Source: three-view drawing plus pictorial views. Frame: mm from the lowest corner of the part. Round coordinates to 2 decimals unless told otherwise and drop trailing zeros. Loops run counter-clockwise (first coordinate to the right, second up) from the corner with the lowest first, then second, coordinate; pieces in that order, holes last. Notation, with made-up numbers: (50, -33) -> (55, -33) arc R20 cw to (55, -28) -> close; hole circle Ø7 at (29, 41). An arc over 180 degrees is marked (long way). Return JSON: item names as keys, results as strings. Group by question number.
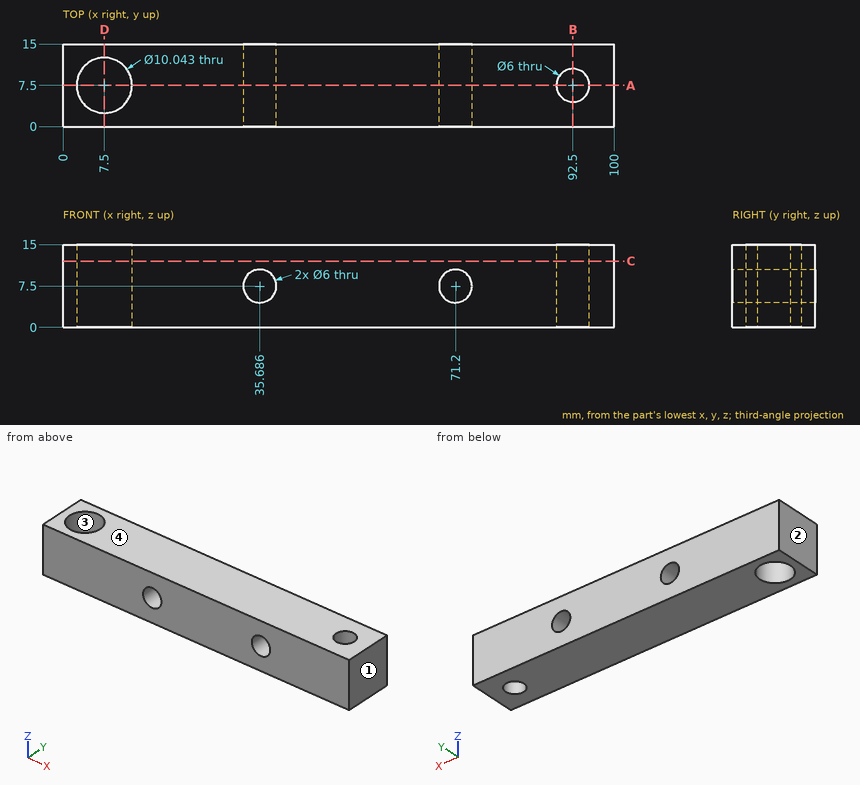
(1) Mould query, pull axis X, two halves, no side actions, for the marked faces 1, 2, 3 and 4. Classes: released by +X, released by -X, zero draft, split by the parting line, or undercut.
(2) Ray query, line 1 (X direction, y = 13, z = 7.75) (1 decimal); line 2 (Y direction, x = 92.5, z = 1.5); line 3 (X direction, y = 5.5, z = 12.5) (1 decimal). Return the intervals inside material, ascending.
(3) Cut plane A-A (y = 7.5). Return loops of the section in (x, z), and give its area (3 significant figures).
(4) Pin query (flat end, axial travel): pin 1 (5.5 mm diameter, centred on x = 71.2, z = 7.5, fed in from +Y). Return the tip coordinate at first contact, or that it passes through.
(5) Cut plane C-C (z = 12). Return loops of the section in (x, y), and give its area (3 significant figures).
(6) Cut plane D-D (x = 7.5). Return loops of the section in (y, z).
(7) Cut plane B-B (x = 92.5). Return loops of the section in (y, z).
Answers follow:
{
 "1": {"face 1": "released by +X", "face 2": "released by -X", "face 3": "undercut", "face 4": "zero draft"},
 "2": {"line 1": "0 to 32.7, 38.7 to 68.2, 74.2 to 100", "line 2": "0 to 4.5, 10.5 to 15", "line 3": "0 to 2.9, 12.1 to 90.3, 94.7 to 100"},
 "3": {"outline": "(0, 0) -> (2.48, 0) -> (2.48, 15) -> (0, 15) -> close; (12.52, 0) -> (89.5, 0) -> (89.5, 15) -> (12.52, 15) -> close; (95.5, 0) -> (100, 0) -> (100, 15) -> (95.5, 15) -> close; hole circle Ø6 at (35.69, 7.5); hole circle Ø6 at (71.2, 7.5)", "area": "1,200 mm^2"},
 "4": {"pin 1": "through"},
 "5": {"outline": "(0, 0) -> (100, 0) -> (100, 15) -> (0, 15) -> close; hole circle Ø10.04 at (7.5, 7.5); hole circle Ø6 at (92.5, 7.5)", "area": "1,390 mm^2"},
 "6": {"outline": "(0, 0) -> (2.48, 0) -> (2.48, 15) -> (0, 15) -> close; (12.52, 0) -> (15, 0) -> (15, 15) -> (12.52, 15) -> close"},
 "7": {"outline": "(0, 0) -> (4.5, 0) -> (4.5, 15) -> (0, 15) -> close; (10.5, 0) -> (15, 0) -> (15, 15) -> (10.5, 15) -> close"}
}
